For this review, take the finished solid that the model builds, in its own axes (mm). A direction names the side the tool comes from. Coordinates: 2 decimals unless noted, no trailing zeros. Order: outer loops, then holes, each group sorted by start corner. A loop starts at its lowest first (then second) coordinate and runs counter-clockwise, first axis right, second up. Notation, with made-up numbers: M 44,-19 L 102,-19 A27 ccw 102,-1 Z; hole C 63.25,65 d7. An arc over 180 degrees is marked long. Use CSV: the item, a comma, the result in double quotes.
```python
from build123d import *

# Parameters (mm, degrees)
BOSS_EXTRUDE1_DEPTH      = 12
BOSS_EXTRUDE1_DEPTH_BACK = 12
SKETCH1_W                = 80
SKETCH1_H                = 20
SKETCH1_R                = 6
SKETCH1_R_2              = 7.5
SKETCH2_W                = 25
SKETCH2_H                = 54
BOSS_EXTRUDE2_DEPTH      = 7
CUT_EXTRUDE1_DEPTH       = 3
MIRROR2_COPY_1_DEPTH     = 3
D_GAGEMENT_M41_D         = 4.5
CUT_EXTRUDE2_DEPTH       = 59.395205283
SKETCH7_W                = 25
SKETCH7_H                = 20
BOSS_EXTRUDE3_DEPTH      = 3
SKETCH8_W                = 25
SKETCH8_H                = 20
BOSS_EXTRUDE4_DEPTH      = 3
CUT_EXTRUDE3_DEPTH       = 59.395205283
CUT_EXTRUDE3_DEPTH_BACK  = 59.395205283
SKETCH10_R               = 5
FILLET1_R                = 3


with BuildPart() as part:
    # Sketch1 → Boss-Extrude1 (new, two sides: drawn at the far end of the back side and taken through both)
    with BuildSketch(Plane.XY.offset(-BOSS_EXTRUDE1_DEPTH_BACK)):
        Rectangle(SKETCH1_W, SKETCH1_H)
        Circle(SKETCH1_R, mode=Mode.SUBTRACT)
        with Locations((30, 0)):
            Circle(SKETCH1_R_2, mode=Mode.SUBTRACT)
        with Locations((-30, 0)):
            Circle(SKETCH1_R_2, mode=Mode.SUBTRACT)
    extrude(amount=BOSS_EXTRUDE1_DEPTH + BOSS_EXTRUDE1_DEPTH_BACK)

    # Sketch2 → Boss-Extrude2 (add)
    with BuildSketch(Plane.XZ.offset(10)):
        with Locations((27.5, 0)):
            Rectangle(SKETCH2_W, SKETCH2_H)
        with Locations((-27.5, 0)):
            Rectangle(SKETCH2_W, SKETCH2_H)
    extrude(amount=BOSS_EXTRUDE2_DEPTH)

    # Sketch3 → Cut-Extrude1 (cut)
    with BuildSketch(Plane(origin=(0, -10, 0), x_dir=(1, 0, 0), z_dir=(0, 1, 0))):
        Polygon((29.520725942, 23.000000033), (25.479274058, 23.000000033), (23.458548116, 19.500000033), (25.479274058, 16.000000033), (29.520725942, 16.000000033), (31.541451884, 19.500000033), align=None)
    cut_extrude1 = extrude(amount=-CUT_EXTRUDE1_DEPTH, mode=Mode.SUBTRACT)

    # Mirror1: Cut-Extrude1 across plane
    add(cut_extrude1.mirror(Plane(origin=(0, 0, 0), x_dir=(0, 0, 1), z_dir=(1, 0, 0))), mode=Mode.SUBTRACT)

    # Mirror2: Cut-Extrude1 across plane
    add(cut_extrude1.mirror(Plane.XY), mode=Mode.SUBTRACT)

    # Mirror2 copy 1 sketch → Mirror2 copy 1 (cut)
    with BuildSketch(Plane(origin=(0, -10, 0), x_dir=(-1, 0, 0), z_dir=(0, 1, 0))):
        Polygon((29.520725942, 23.000000033), (25.479274058, 23.000000033), (23.458548116, 19.500000033), (25.479274058, 16.000000033), (29.520725942, 16.000000033), (31.541451884, 19.500000033), align=None)
    extrude(amount=-MIRROR2_COPY_1_DEPTH, mode=Mode.SUBTRACT)

    # Dégagement M41 (through all)
    with Locations(Plane(origin=(0, -13, 0), x_dir=(1, 0, 0), z_dir=(0, 1, 0))):
        with Locations((27.5, 19.5), (27.5, -19.5), (-27.5, -19.5), (-27.5, 19.5)):
            Hole(D_GAGEMENT_M41_D / 2)

    # Sketch6 → Cut-Extrude2 (cut, through all)
    with BuildSketch(Plane(origin=(0, 0, -12), x_dir=(-1, 0, 0), z_dir=(0, 0, -1))):
        with BuildLine():
            Line((-30, 7.5), (-40, 7.5))
            Line((-40, 7.5), (-40, -7.5))
            Line((-40, -7.5), (-30, -7.5))
            ThreePointArc((-30, -7.5), (-37.5, 0), (-30, 7.5))
        make_face()
    cut_extrude2 = extrude(amount=-CUT_EXTRUDE2_DEPTH, mode=Mode.SUBTRACT)

    # Mirror3: Cut-Extrude2 across plane
    add(cut_extrude2.mirror(Plane(origin=(0, 0, 0), x_dir=(0, 0, 1), z_dir=(1, 0, 0))), mode=Mode.SUBTRACT)

    # Sketch7 → Boss-Extrude3 (add)
    with BuildSketch(Plane(origin=(0, 0, -12), x_dir=(-1, 0, 0), z_dir=(0, 0, -1))):
        with Locations((-27.5, 0)):
            Rectangle(SKETCH7_W, SKETCH7_H)
        with Locations((27.5, 0)):
            Rectangle(SKETCH7_W, SKETCH7_H)
    extrude(amount=BOSS_EXTRUDE3_DEPTH)

    # Sketch8 → Boss-Extrude4 (add)
    with BuildSketch(Plane.XY.offset(12)):
        with Locations((27.5, 0)):
            Rectangle(SKETCH8_W, SKETCH8_H)
        with Locations((-27.5, 0)):
            Rectangle(SKETCH8_W, SKETCH8_H)
    extrude(amount=BOSS_EXTRUDE4_DEPTH)

    # Sketch10 → Cut-Extrude3 (cut, two sides: drawn at the far end of the back side and taken through both)
    with BuildSketch(Plane.XY.offset(-12).offset(-CUT_EXTRUDE3_DEPTH_BACK)):
        with Locations((30, 0)):
            Circle(SKETCH10_R)
        with Locations((-30, 0)):
            Circle(SKETCH10_R)
    extrude(amount=CUT_EXTRUDE3_DEPTH + CUT_EXTRUDE3_DEPTH_BACK, mode=Mode.SUBTRACT)

    # Fillet1
    fillet1_edges = [part.edges().sort_by_distance(p)[0] for p in [
        (15, -10, 0),
        (-15, -10, 0),
        (-15, 0, -12),
        (15, 0, -12),
        (-15, 0, 12),
        (15, 0, 12),
    ]]
    fillet(fillet1_edges, radius=FILLET1_R - 0.0001)  # a hair under: the kernel refuses the full size


solid = part.part
```
Item 1: Add section A-A on z = -14. State the section outline as (x, y) points.
Solutions:
outline,"M -40,-17 L -15,-17 L -15,-13 A3 cw -14.83,-12 L -14.83,10 L -40,10 Z; M 14.83,-12 A3 cw 15,-13 L 15,-17 L 40,-17 L 40,10 L 14.83,10 Z; hole C -30,0 d10; hole C 30,0 d10"
Item 2: Add section D-D on x = -3. State the section outline as (y, z) points.
Solutions:
outline,"M -10,-12 L -5.2,-12 L -5.2,12 L -10,12 Z; M 5.2,-12 L 10,-12 L 10,12 L 5.2,12 Z"
Item 3: To check wall thickness, follow line 1 along Z through (x, y) = (-27.5, -15.35); line 2 along X through (y, z) = (-14.1, -19.5); line 3 along Z through (x, y) = (-36.5, -0.5). State the ranges of each line that lie inside material, in increasing order. Write a range as [from, to].
Solutions:
line 1,"[-27, -21.75], [-17.25, 17.25], [21.75, 27]"
line 2,"[-40, -29.75], [-25.25, -15], [15, 25.25], [29.75, 40]"
line 3,"[-15, -12], [12, 15]"
Item 4: For faces 4 (the face through (-28, -10, 24)), 5 (the face through (-35.3, 0.1, 12)), 6 (the face through (25, 0, 13)), 7 (the face through (-27, -11, 16)), list the 3-axis set-ups (+Z, -Z, +X, -X, +Y, -Y) from which the entire face can be reached by the end or side of a thin tool; tool diameter is ignored.
Solutions:
face 4,"+Z, +X, -X, +Y"
face 5,"-X"
face 6,"+Z, -Z"
face 7,"+Y"
Item 5: Add section B-B on x = 18. State the section outline as (y, z) points, and give its area (3 significant figures).
Solutions:
outline,"M -17,-27 L -10,-27 L -10,-15 L 10,-15 L 10,15 L -10,15 L -10,27 L -17,27 Z"
area,"978 mm^2"
Item 6: Add section C-C on z = -4.5. State the section outline as (x, y) points.
Solutions:
outline,"M -40,-17 L -15,-17 L -15,-13 A3 cw -12,-10 L 12,-10 A3 cw 15,-13 L 15,-17 L 40,-17 L 40,-7.5 L 30,-7.5 A7.5 cw 30,7.5 L 40,7.5 L 40,10 L -40,10 L -40,7.5 L -30,7.5 A7.5 cw -30,-7.5 L -40,-7.5 Z; hole C 0,0 d12"
Item 7: Clearance check with flat-ended pins moving along their axes: pin 1 Ø14 at (x, y) = (0, 0) entering from +Z; pin 2 Ø10 at (x, y) = (26.5, -1.5) entering from +Z; pin 3 Ø6 at (x, y) = (-4.5, -2.5) entering from -Z; pin 4 Ø3 at (y, z) = (-7, -6) entering from -X. State where each tip first meets the part, or that it passes through.
Solutions:
pin 1,"z = 12"
pin 2,"z = 15"
pin 3,"z = -12"
pin 4,"x = -40"
Item 8: Draft analysis for pull direction Z (two halves, no side actions). For faces 1 (the face through (40, -10, 0)), 2 (the face through (24.455, -11.479, -17.775)), 3 (the face through (25, 2, -15)), state which applies: released by +Z, released by -Z, zero draft, split by the parting line, or undercut.
Solutions:
face 1,"zero draft"
face 2,"undercut"
face 3,"released by -Z"
